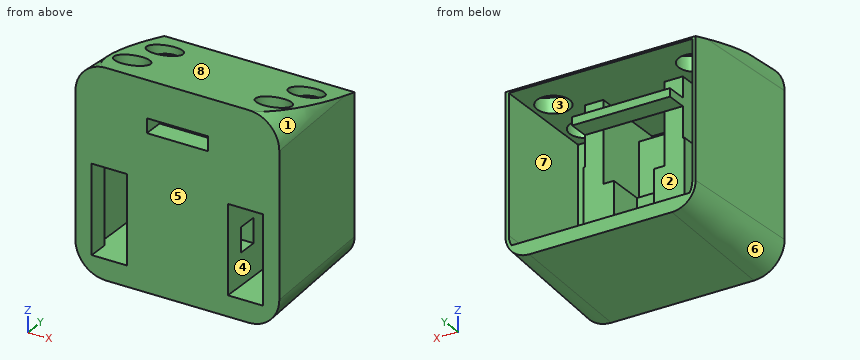
from build123d import *

# Parameters (mm, degrees)
BOSS_EXTRUDE1_DEPTH  = 10
SKETCH2_W            = 17.2
SKETCH2_H            = 43
CUT_EXTRUDE1_DEPTH   = 72.414284285
SKETCH3_W            = 90
SKETCH3_H            = 34
SKETCH3_W_2          = 80
SKETCH3_H_2          = 24
BOSS_EXTRUDE3_DEPTH  = 15
SKETCH4_W            = 49.6
SKETCH4_H            = 5
BOSS_EXTRUDE4_DEPTH  = 10
SKETCH5_W            = 15
SKETCH5_H            = 22
BOSS_EXTRUDE5_DEPTH  = 5
SKETCH6_W            = 90
SKETCH6_H            = 77
BOSS_EXTRUDE6_DEPTH  = 15
BOSS_EXTRUDE8_DEPTH  = 39
CHAMFER1_SIZE        = 64
CHAMFER1_SIZE_2      = 3.354097874
CHAMFER3_SIZE        = 64
CHAMFER3_SIZE_2      = 13.775745352
CUT_EXTRUDE6_DEPTH   = 2.5
CUT_EXTRUDE8_DEPTH   = 15
CUT_EXTRUDE9_DEPTH   = 15
SKETCH22_W           = 30
SKETCH22_H           = 7
CUT_EXTRUDE10_DEPTH  = 10
SKETCH25_R           = 8
CUT_EXTRUDE19_DEPTH  = 116.41230437
SKETCH29_W           = 9
SKETCH29_H           = 29
BOSS_EXTRUDE10_DEPTH = 28
SKETCH31_W           = 49.6
SKETCH31_H           = 13
BOSS_EXTRUDE12_DEPTH = 28
SKETCH30_W           = 49.6
SKETCH30_H           = 4
SKETCH30_W_2         = 48
BOSS_EXTRUDE11_DEPTH = 10
SKETCH33_W           = 15
SKETCH33_H           = 19.5
BOSS_EXTRUDE13_DEPTH = 13
SKETCH23_W           = 30
SKETCH23_H           = 28.995403325
CUT_EXTRUDE17_DEPTH  = 5
SKETCH34_W           = 9.8
SKETCH34_H           = 10.5
BOSS_EXTRUDE14_DEPTH = 28
SKETCH35_W           = 30
SKETCH35_H           = 10.5
CUT_EXTRUDE22_DEPTH  = 5
SKETCH37_W           = 30
SKETCH37_H           = 32.5
BOSS_EXTRUDE15_DEPTH = 5


with BuildPart() as part:
    # Sketch1 → Boss-Extrude1 (new body)
    with BuildSketch(Plane(origin=(0, 0, 0), x_dir=(1, 0, 0), z_dir=(0, 1, 0))):
        with BuildLine():
            Line((-35, 50), (35, 50))
            ThreePointArc((35, 50), (45.606601718, 45.606601718), (50, 35))
            Line((50, 35), (50, -35))
            ThreePointArc((50, -35), (45.606601718, -45.606601718), (35, -50))
            Line((35, -50), (-35, -50))
            ThreePointArc((-35, -50), (-45.606601718, -45.606601718), (-50, -35))
            Line((-50, -35), (-50, 35))
            ThreePointArc((-50, 35), (-45.606601718, 45.606601718), (-35, 50))
        make_face()
    extrude(amount=BOSS_EXTRUDE1_DEPTH)

    # Sketch2 → Cut-Extrude1 (cut, through all)
    with BuildSketch(Plane(origin=(0, 10, 0), x_dir=(1, 0, 0), z_dir=(0, 1, 0))):
        with Locations((-33.4, 18.5)):
            Rectangle(SKETCH2_W, SKETCH2_H)
        with Locations((33.4, 18.5)):
            Rectangle(SKETCH2_W, SKETCH2_H)
    extrude(amount=-CUT_EXTRUDE1_DEPTH, mode=Mode.SUBTRACT)

    # Sketch3 → Boss-Extrude3 (add)
    with BuildSketch(Plane(origin=(0, 10, 0), x_dir=(1, 0, 0), z_dir=(0, 1, 0))):
        with Locations((0, -20)):
            Rectangle(SKETCH3_W, SKETCH3_H)
        with Locations((0, -20)):
            Rectangle(SKETCH3_W_2, SKETCH3_H_2, mode=Mode.SUBTRACT)
    extrude(amount=BOSS_EXTRUDE3_DEPTH)

    # Sketch4 → Boss-Extrude4 (add)
    with BuildSketch(Plane(origin=(0, 10, 0), x_dir=(1, 0, 0), z_dir=(0, 1, 0))):
        with Locations((0, 10)):
            Rectangle(SKETCH4_W, SKETCH4_H)
        with Locations((0, 27)):
            Rectangle(SKETCH4_W, SKETCH4_H)
    extrude(amount=BOSS_EXTRUDE4_DEPTH)

    # Sketch5 → Boss-Extrude5 (add)
    with BuildSketch(Plane(origin=(0, 20, 0), x_dir=(1, 0, 0), z_dir=(0, 1, 0))):
        with Locations((-17.3, 18.5)):
            Rectangle(SKETCH5_W, SKETCH5_H)
        with Locations((17.3, 18.5)):
            Rectangle(SKETCH5_W, SKETCH5_H)
    extrude(amount=BOSS_EXTRUDE5_DEPTH)

    # Sketch6 → Boss-Extrude6 (add)
    with BuildSketch(Plane(origin=(0, 10, 0), x_dir=(1, 0, 0), z_dir=(0, 1, 0))):
        with BuildLine():
            Line((-50, 35), (-50, -35))
            ThreePointArc((-50, -35), (-45.606601718, -45.606601718), (-35, -50))
            Line((-35, -50), (35, -50))
            ThreePointArc((35, -50), (45.606601718, -45.606601718), (50, -35))
            Line((50, -35), (50, 35))
            ThreePointArc((50, 35), (45.606601718, 45.606601718), (35, 50))
            Line((35, 50), (-35, 50))
            ThreePointArc((-35, 50), (-45.606601718, 45.606601718), (-50, 35))
        make_face()
        with Locations((0, 1.5)):
            Rectangle(SKETCH6_W, SKETCH6_H, mode=Mode.SUBTRACT)
    extrude(amount=BOSS_EXTRUDE6_DEPTH)

    # Sketch9 → Boss-Extrude8 (add)
    with BuildSketch(Plane(origin=(0, 25, 0), x_dir=(1, 0, 0), z_dir=(0, 1, 0))):
        with BuildLine():
            Line((-50, 35), (-50, -35))
            ThreePointArc((-50, -35), (-45.606601718, -45.606601718), (-35, -50))
            Line((-35, -50), (35, -50))
            ThreePointArc((35, -50), (45.606601718, -45.606601718), (50, -35))
            Line((50, -35), (50, 35))
            ThreePointArc((50, 35), (45.606601718, 45.606601718), (35, 50))
            Line((35, 50), (-35, 50))
            ThreePointArc((-35, 50), (-45.606601718, 45.606601718), (-50, 35))
        make_face()
        with BuildLine():
            Line((-45, 35), (-45, -32))
            Line((-45, -32), (45, -32))
            Line((45, -32), (45, 35))
            ThreePointArc((45, 35), (44.659258263, 37.588190451), (43.660254038, 40))
            Line((43.660254038, 40), (-43.660254038, 40))
            ThreePointArc((-43.660254038, 40), (-44.659258263, 37.588190451), (-45, 35))
        make_face(mode=Mode.SUBTRACT)
    extrude(amount=BOSS_EXTRUDE8_DEPTH)

    # Chamfer1
    # the kernel refuses this chamfer: 64, 3.354097874 mm, written as the material it takes off along each edge
    with BuildSketch(Plane(origin=(-35, 64, 50), x_dir=(0, -0.9999979738662979, 0.002013023422382214), z_dir=(1, 0, 0)), Plane(origin=(50, 64, 35), x_dir=(0.002013023422382214, -0.9999979738662979, 0), z_dir=(0, 0, -1)), Plane(origin=(-50, 64, -35), x_dir=(-0.002013023422382214, -0.9999979738662979, 0), z_dir=(0, 0, 1)), Plane(origin=(35, 64, -50), x_dir=(0, -0.9999979738662979, -0.002013023422382214), z_dir=(-1, 0, 0))) as chamfer1_piece_1:
        Polygon((CHAMFER1_SIZE * 0.999997973866, CHAMFER1_SIZE * 0.00201302342238), (-CHAMFER1_SIZE_2 * 0.00201302342245, CHAMFER1_SIZE_2 * 0.9999979739), (0, 0), align=None)
    extrude(amount=70, mode=Mode.SUBTRACT)
    with BuildSketch(Plane(origin=(35, 64, 35), x_dir=(0, 0, 1), z_dir=(-1, 0, 0))) as chamfer1_piece_2:
        Polygon((15, -CHAMFER1_SIZE), (15 - CHAMFER1_SIZE_2, 0), (15, 0), align=None)
    revolve(axis=Axis((35, 64, 35), (0, 1, 0)), revolution_arc=90, mode=Mode.SUBTRACT)
    with BuildSketch(Plane(origin=(-35, 64, 35), x_dir=(-1, 0, 0), z_dir=(0, 0, -1))) as chamfer1_piece_3:
        Polygon((15, -CHAMFER1_SIZE), (15 - CHAMFER1_SIZE_2, 0), (15, 0), align=None)
    revolve(axis=Axis((-35, 64, 35), (0, 1, 0)), revolution_arc=90, mode=Mode.SUBTRACT)
    with BuildSketch(Plane(origin=(35, 64, -35), x_dir=(1, 0, 0), z_dir=(0, 0, 1))) as chamfer1_piece_4:
        Polygon((15, -CHAMFER1_SIZE), (15 - CHAMFER1_SIZE_2, 0), (15, 0), align=None)
    revolve(axis=Axis((35, 64, -35), (0, 1, 0)), revolution_arc=90, mode=Mode.SUBTRACT)
    with BuildSketch(Plane(origin=(-35, 64, -35), x_dir=(0, 0, -1), z_dir=(1, 0, 0))) as chamfer1_piece_5:
        Polygon((15 - CHAMFER1_SIZE_2, 0), (15, -CHAMFER1_SIZE), (15, 0), align=None)
    revolve(axis=Axis((-35, 64, -35), (0, 1, 0)), revolution_arc=90, mode=Mode.SUBTRACT)

    # Chamfer3
    # the kernel refuses this chamfer: 64, 13.775745352 mm, written as the material it takes off along each edge
    with BuildSketch(Plane(origin=(-201.265469314, 64, 46.645902126), x_dir=(0, -0.9981787050157903, 0.06032638604292662), z_dir=(1, 0, 0))) as chamfer3_piece_1:
        Polygon((CHAMFER3_SIZE * 0.999967974892, CHAMFER3_SIZE * 0.00800307379952), (-CHAMFER3_SIZE_2 * 0.060326386045, CHAMFER3_SIZE_2 * 0.99817870505), (0, 0), align=None)
    extrude(amount=402.530938629, mode=Mode.SUBTRACT)

    # Sketch17 → Cut-Extrude6 (cut)
    with BuildSketch(Plane(origin=(0, 0, -29.5), x_dir=(-1, 0, 0), z_dir=(0, 0, -1))):
        Polygon((-24.8, 10), (24.8, 10), (24.8, 25), (9.8, 25), (9.8, 20), (-9.8, 20), (-9.8, 25), (-24.8, 25), align=None)
    extrude(amount=-CUT_EXTRUDE6_DEPTH, mode=Mode.SUBTRACT)

    # Sketch20 → Cut-Extrude8 (cut)
    with BuildSketch(Plane.XZ.offset(-25)):
        with BuildLine():
            Line((-45, -35), (-45, -40))
            Line((-45, -40), (-43.660254038, -40))
            ThreePointArc((-43.660254038, -40), (-44.659258263, -37.588190451), (-45, -35))
        make_face()
        with BuildLine():
            Line((45, -40), (45, -35))
            ThreePointArc((45, -35), (44.659258263, -37.588190451), (43.660254038, -40))
            Line((43.660254038, -40), (45, -40))
        make_face()
    extrude(amount=-CUT_EXTRUDE8_DEPTH, mode=Mode.SUBTRACT)

    # Sketch21 → Cut-Extrude9 (cut)
    with BuildSketch(Plane(origin=(0, 25, 0), x_dir=(1, 0, 0), z_dir=(0, 1, 0))):
        Polygon((40, -8), (40, -32), (45, -32), (45, -3), (-45, -3), (-45, -32), (-40, -32), (-40, -8), align=None)
    extrude(amount=-CUT_EXTRUDE9_DEPTH, mode=Mode.SUBTRACT)

    # Sketch22 → Cut-Extrude10 (cut)
    with BuildSketch(Plane.XZ):
        with Locations((0, 28.5)):
            Rectangle(SKETCH22_W, SKETCH22_H)
    extrude(amount=-CUT_EXTRUDE10_DEPTH, mode=Mode.SUBTRACT)

    # Sketch25 → Cut-Extrude19 (cut, through all)
    with BuildSketch(Plane(origin=(0, 0, 32), x_dir=(-1, 0, 0), z_dir=(0, 0, -1))):
        with Locations((-34.75, 45.5)):
            Circle(SKETCH25_R)
        with Locations((34.75, 45.5)):
            Circle(SKETCH25_R)
        with Locations((-34.75, 20)):
            Circle(SKETCH25_R)
        with Locations((34.75, 20)):
            Circle(SKETCH25_R)
    extrude(amount=-CUT_EXTRUDE19_DEPTH, mode=Mode.SUBTRACT)

    # Sketch29 → Boss-Extrude10 (add)
    with BuildSketch(Plane(origin=(0, 10, 0), x_dir=(1, 0, 0), z_dir=(0, 1, 0))):
        with Locations((-19.5, -17.5)):
            Rectangle(SKETCH29_W, SKETCH29_H)
        with Locations((19.5, -17.5)):
            Rectangle(SKETCH29_W, SKETCH29_H)
    extrude(amount=BOSS_EXTRUDE10_DEPTH)

    # Sketch31 → Boss-Extrude12 (add)
    with BuildSketch(Plane(origin=(0, 10, 0), x_dir=(1, 0, 0), z_dir=(0, 1, 0))):
        with Locations((0, 33.5)):
            Rectangle(SKETCH31_W, SKETCH31_H)
    extrude(amount=BOSS_EXTRUDE12_DEPTH)

    # Sketch30 → Boss-Extrude11 (add)
    with BuildSketch(Plane(origin=(0, 38, 0), x_dir=(1, 0, 0), z_dir=(0, 1, 0))):
        with Locations((0, 38)):
            Rectangle(SKETCH30_W, SKETCH30_H)
        with Locations((0, -20)):
            Rectangle(SKETCH30_W_2, SKETCH30_H)
    extrude(amount=BOSS_EXTRUDE11_DEPTH)

    # Sketch33 → Boss-Extrude13 (add)
    with BuildSketch(Plane(origin=(0, 25, 0), x_dir=(1, 0, 0), z_dir=(0, 1, 0))):
        with Locations((17.3, 17.25)):
            Rectangle(SKETCH33_W, SKETCH33_H)
        with Locations((-17.3, 17.25)):
            Rectangle(SKETCH33_W, SKETCH33_H)
    extrude(amount=BOSS_EXTRUDE13_DEPTH)

    # Sketch23 → Cut-Extrude17 (cut)
    with BuildSketch(Plane(origin=(0, 10, 0), x_dir=(1, 0, 0), z_dir=(0, 1, 0))):
        with Locations((0, -17.497701662)):
            Rectangle(SKETCH23_W, SKETCH23_H)
    extrude(amount=-CUT_EXTRUDE17_DEPTH, mode=Mode.SUBTRACT)

    # Sketch34 → Boss-Extrude14 (add)
    with BuildSketch(Plane(origin=(0, 10, 0), x_dir=(1, 0, 0), z_dir=(0, 1, 0))):
        with Locations((-19.9, 2.25)):
            Rectangle(SKETCH34_W, SKETCH34_H)
        with Locations((19.9, 2.25)):
            Rectangle(SKETCH34_W, SKETCH34_H)
    extrude(amount=BOSS_EXTRUDE14_DEPTH)

    # Sketch35 → Cut-Extrude22 (cut)
    with BuildSketch(Plane(origin=(0, 10, 0), x_dir=(1, 0, 0), z_dir=(0, 1, 0))):
        with Locations((0, 2.25)):
            Rectangle(SKETCH35_W, SKETCH35_H)
    extrude(amount=-CUT_EXTRUDE22_DEPTH, mode=Mode.SUBTRACT)

    # Sketch37 → Boss-Extrude15 (add)
    with BuildSketch(Plane(origin=(0, 5, 0), x_dir=(1, 0, 0), z_dir=(0, 1, 0))):
        with Locations((0, -8.75)):
            Rectangle(SKETCH37_W, SKETCH37_H)
    extrude(amount=BOSS_EXTRUDE15_DEPTH)


solid = part.part
Input: part model. Units: mm. Frame: model coordinates. Face numbers are marked on the shaded views. A direction names the side the tool comes from. Coordinates: 2 decimals unless noted, no trailing zeros. Order: outer loops, then holes, each group sorted by start corner. A loop starts at its lowest first (then second) coordinate and runs counter-clockwise, first axis right, second up. Notation, with made-up numbers: M 10,53.5 L 21,53.5 A13 cw 21,74.5 Z; hole C 1.5,48 d3. An arc over 180 degrees is marked long. Write item = value, one per line. Start each with the question number.
(1) Section A-A on z = -30. Output: boundary loops of the cut face in (x, y), and give its area (3 significant figures).
(2) Section B-B on x = -19. Output: boundary loops of the cut face in (y, z), and give its area (3 significant figures).
(3) First-contact query: P1, Ø10.5, axis at x = -38.5, z = 13.5, coming from the +Y side; P2, Ø9.5, axis at x = -34.75, y = 20, coming from the -Z side; P3, Ø1.5, axis at y = 35.5, z = 24, coming from the +X side. Flat tips, straight axial feed; report the tip coordinate or a pass-through.
(4) Section C-C on z = 11.5. Output: boundary loops of the cut face in (x, y).
(5) Pull-direction query (Z, two-part tool) for the marked faces 6, 7 and 8; classes: released by +Z, released by -Z, zero draft, split by the parting line, or undercut.
(6) Section D-D on x = -4. Output: boundary loops of the cut face in (y, z), and give its area (3 significant figures).
(7) Reachability of the marked faces 1, 2, 3, 4 and 5 from +Z, -Z, +X, -X, +Y, -Y: full face, straight path, thin tool, end or side. Return the list, or none.
(8) Line query: line 1 along Y through (x, z) = (-19, -14); line 2 along Y through (x, z) = (-34.75, 38.5); line 3 along X through (y, z) = (26, 16.5). Output: solid intervals per line, ascending. Write a range as [from, to].
Result set:
q1.outline = M -50,0 L -42,0 L -42,10 L -45,10 L -45,64 L -46.65,64 Z; M -24.8,0 L 24.8,0 L 24.8,38 L -24.8,38 Z; M 42,0 L 50,0 L 46.65,64 L 45,64 L 45,10 L 42,10 Z
q1.area = 2,370 mm²
q2.outline = M 0,-50 L 64,-46.65 L 64,-40 L 48,-40 L 48,-36 L 38,-36 L 38,18 L 48,18 L 48,22 L 38,22 L 38,32 L 64,32 L 64,32.87 L 0.09,50 L 0,50 Z; hole M 10,-24.5 L 20,-24.5 L 20,-12.5 L 10,-12.5 Z
q2.area = 3,830 mm²
q3.P1 = 10
q3.P2 = -49.2
q3.P3 = 48.18
q4.outline = M -50,0 L 50,0 L 46.65,64 L 45,64 L 45,10 L 24,10 L 24,38 L 15,38 L 15,10 L -15,10 L -15,38 L -24,38 L -24,10 L -45,10 L -45,64 L -46.65,64 Z
q5.face_6 = released by -Z
q5.face_7 = undercut
q5.face_8 = released by +Z
q6.outline = M 0,-50 L 64,-46.65 L 64,-40 L 48,-40 L 48,-36 L 38,-36 L 38,-27 L 20,-27 L 20,-24.5 L 10,-24.5 L 10,-12.5 L 20,-12.5 L 20,-7.5 L 10,-7.5 L 10,25 L 0,25 Z; M 0,32 L 64,32 L 64,32.87 L 0.09,50 L 0,50 Z; M 38,18 L 48,18 L 48,22 L 38,22 Z
q6.area = 2,310 mm²
q7.face_1 = +Z, +X, +Y
q7.face_2 = +Y
q7.face_3 = +Z
q7.face_4 = +Y, -Y
q7.face_5 = +Z, -Z, +X, -X, -Y
q8.line_1 = [0, 10], [20, 38]
q8.line_2 = [0, 12], [28, 37.5]
q8.line_3 = [-48.64, -45], [-24, -15], [15, 24], [45, 48.64]
